Read the model definition and answer for the solid it produces. Units are mm, in the model's axes. A direction names the side the tool comes from. Give positions to 0.01 mm unless a question says otherwise; leave off trailing zeros. Loops run counter-clockwise (first coordinate to the right, second up) from the corner with the lowest first, then second, coordinate; pieces in that order, holes last. Notation, with made-up numbers: (79.25, 67) - (88.25, 67) arc R21 cw to (88.25, 102) - close; hole circle Ø9 at (-23.75, 25.5). An arc over 180 degrees is marked (long way). Use a Markdown table: item, result. Add a question column.
Item 1: A cutting plane is placed at A-A (x = 19.5). Determine the outline of the cut face in (y, z).
Item 2: A cutting plane is placed at B-B (z = 9). Determine the outline of the cut face in (x, y).
Item 3: For a pull along Y with two mould halves and no side action, classify faces 1 (the face through (30, 12, 10)), 2 (the face through (22.395, 20.07, 17.465)), 3 (the face through (18, 0, 8)) as +Y half, -Y half, draft (parallel to the pull), parting line (faces both ways), or undercut.
Item 4: Which of the six approach directions +Z, -Z, +X, -X, +Y, -Y give full straight-line access (tool end or side, diameter ignored) to faces 4 (the face through (7, 8, 10)), 5 (the face through (11, 15, 5)), 6 (the face through (15, 8, 0))?
Item 5: Consider probe 1 along Z at (x, y) = (14, 14.5); probe 2 along X at (y, z) = (2, 16.5); probe 3 along Y at (x, z) = (13.75, 9.25). Determine where each line is inside the solid, lowest interval first. Write a range as [from, to].
Item 6: A cutting plane is placed at D-D (x = 25.5). Determine the outline of the cut face in (y, z).
Item 7: Each of these flat-tipped pins is pushed along its axis until it touches: P1, Ø5, axis at y = 21, z = 12.5, coming from the -X side; P2, Ø3, axis at x = 11.5, z = 4, coming from the +Y side; P3, Ø5, axis at y = 20.5, z = 7, coming from the -X side. Where does it stop, or does it pass through?
Item 8: A cutting plane is placed at C-C (y = 12.5). Determine the outline of the cut face in (x, z), plus the area to 3 significant figures.
from build123d import *

# Parameters (mm, degrees)
SKETCH1_W           = 30
SKETCH1_H           = 25
BOSS_EXTRUDE1_DEPTH = 20
SKETCH2_W           = 15
SKETCH2_H           = 25
CUT_EXTRUDE1_DEPTH  = 10
SKETCH3_W           = 15
SKETCH3_H           = 10
CUT_EXTRUDE2_DEPTH  = 10
CUT_EXTRUDE3_DEPTH  = 20
CUT_EXTRUDE4_DEPTH  = 10


with BuildPart() as part:
    # Sketch1 → Boss-Extrude1 (new body)
    with BuildSketch(Plane.XY):
        with Locations((15, 12.5)):
            Rectangle(SKETCH1_W, SKETCH1_H)
    extrude(amount=BOSS_EXTRUDE1_DEPTH)

    # Sketch2 → Cut-Extrude1 (cut)
    with BuildSketch(Plane.XY.offset(20)):
        with Locations((7.5, 12.5)):
            Rectangle(SKETCH2_W, SKETCH2_H)
    extrude(amount=-CUT_EXTRUDE1_DEPTH, mode=Mode.SUBTRACT)

    # Sketch3 → Cut-Extrude2 (cut)
    with BuildSketch(Plane.XY.offset(10)):
        with Locations((7.5, 20)):
            Rectangle(SKETCH3_W, SKETCH3_H)
    extrude(amount=-CUT_EXTRUDE2_DEPTH, mode=Mode.SUBTRACT)

    # Sketch4 → Cut-Extrude3 (cut)
    with BuildSketch(Plane.ZY.offset(-15)):
        Polygon((15, 25), (20, 15), (20, 25), align=None)
    extrude(amount=-CUT_EXTRUDE3_DEPTH, mode=Mode.SUBTRACT)

    # Sketch5 → Cut-Extrude4 (cut)
    with BuildSketch(Plane(origin=(0, 25, 0), x_dir=(1, 0, 0), z_dir=(0, 1, 0))):
        Polygon((15, -10), (30, 0), (15, 0), align=None)
    extrude(amount=-CUT_EXTRUDE4_DEPTH, mode=Mode.SUBTRACT)


solid = part.part
Geometry says:
| question | item | result |
|---|---|---|
| 1 | outline | (0, 0) - (15, 0) - (15, 7) - (25, 7) - (25, 15) - (15, 20) - (0, 20) - close |
| 2 | outline | (0, 0) - (30, 0) - (30, 25) - (16.5, 25) - (16.5, 15) - (0, 15) - close |
| 3 | face 1 | draft |
| 3 | face 2 | +Y half |
| 3 | face 3 | -Y half |
| 4 | face 4 | +Z, -X, +Y, -Y |
| 4 | face 5 | -Z, -X, +Y |
| 4 | face 6 | -Z, +X, -X, +Y, -Y |
| 5 | probe 1 | [0, 10] |
| 5 | probe 2 | [15, 30] |
| 5 | probe 3 | [0, 15] |
| 6 | outline | (0, 0) - (15, 0) - (15, 3) - (25, 3) - (25, 15) - (15, 20) - (0, 20) - close |
| 7 | P1 | x = 15 |
| 7 | P2 | y = 15 |
| 7 | P3 | x = 15.75 |
| 8 | outline | (0, 0) - (30, 0) - (30, 20) - (15, 20) - (15, 10) - (0, 10) - close |
| 8 | area | 450 mm² |
